from build123d import *

# Parameters (mm, degrees)
SKETCH1_R           = 16
BOSS_EXTRUDE1_DEPTH = 100
SKETCH2_R           = 3
BOSS_EXTRUDE2_DEPTH = 15
CIRPATTERN1_COUNT   = 4


with BuildPart() as part:
    # Sketch1 → Boss-Extrude1 (new body)
    with BuildSketch(Plane.XY):
        Circle(SKETCH1_R)
    extrude(amount=BOSS_EXTRUDE1_DEPTH)

    # Sketch2 → Boss-Extrude2 (add)
    with BuildSketch(Plane.XY.offset(100)):
        Circle(SKETCH2_R)
    extrude(amount=BOSS_EXTRUDE2_DEPTH)

    # Sketch6 → M3.5x0.6 Tapped Hole1 (revolve, cut)
    with BuildSketch(Plane(origin=(0, 13, 100), x_dir=(0, -1, 0), z_dir=(1, 0, 0))):
        Polygon((0, 0), (0, 9.761247898), (1.45, 8.89), (1.45, 0), align=None)
    m3_5x0_6_tapped_hole1 = revolve(axis=Axis((0, 13, 106.35), (0, 0, -1)), mode=Mode.SUBTRACT)

    # CirPattern1: M3.5x0.6 Tapped Hole1 ×4 about axis
    cirpattern1_axis = Axis((0, 0, 0), (0, 0, 1))
    for i in range(1, CIRPATTERN1_COUNT):
        add(m3_5x0_6_tapped_hole1.rotate(cirpattern1_axis, i * 360 / CIRPATTERN1_COUNT), mode=Mode.SUBTRACT)


solid = part.part
Geometry: final body of the model. Coordinates: model frame, mm. A direction names the side the tool comes from. Coordinates: 2 decimals unless noted, no trailing zeros. Loops run counter-clockwise (first coordinate to the right, second up) from the corner with the lowest first, then second, coordinate; pieces in that order, holes last. Notation, with made-up numbers: (-39, -30.5) - (-25, -30.5) arc R19 ccw to (-25, -26.5) - close; hole circle Ø6 at (-25.5, -22). An arc over 180 degrees is marked (long way). Put each result on its own line as item: value. Start each with the question number.
Q1. Cut plane D-D, the plane z = 105.5. Return loops of the section in (x, y), and give its area (3 significant figures).
Q2. Line query: line 1 (Z direction, x = -10, y = -2); line 2 (Y direction, x = 13, z = 94.5). Output: solid intervals per line, ascending.
Q3. Pull-direction query (X, two-part tool) for faces 1 (the conical face through (-13.25, -0.01, 90.39)), 2 (the cylindrical face through (-3, 0, 107)), 3 (the flat face through (0, 0, 0)); classes: released by +X, released by -X, zero draft, split by the parting line, or undercut.
Q4. Cut plane A-A, the plane z = 35. Return loops of the section in (x, y).
Q5. Cut plane B-B, the plane x = 6. Return loops of the section in (y, z).
Q6. Cut plane C-C, the plane y = 5. Return loops of the section in (x, z), and give its area (3 significant figures).
Q7. Pin query (flat end, axial travel): pin 1 Ø10 at (y, z) = (8.5, 29.5) entering from -X; pin 2 Ø8 at (x, z) = (-11.5, 96.5) entering from -Y; pin 3 Ø5 at (y, z) = (-10.5, 87.5) entering from -X. Return the tip coordinate at first contact, or that it passes through.
Q8. Set-up query: faces 4 (the cylindrical face through (0.98, -14.07, 95.62)), 5 (the flat face through (0, 0, 115)). Return all of +Z, -Z, +X, -X, +Y, -Y with unobstructed straight access to the full face (end or side cutting, diameter ignored); none if empty.
Filled sheet:
1. outline: circle Ø6 at (0, 0)
1. area: 28.3 mm²
2. line 1: 0 to 100
2. line 2: -9.33 to -1.45, 1.45 to 9.33
3. face 1: undercut
3. face 2: split by the parting line
3. face 3: zero draft
4. outline: circle Ø32 at (0, 0)
5. outline: (-14.83, 0) - (14.83, 0) - (14.83, 100) - (-14.83, 100) - close
6. outline: (-15.2, 0) - (15.2, 0) - (15.2, 100) - (-15.2, 100) - close
6. area: 3,040 mm²
7. pin 1: x = -15.61
7. pin 2: y = -14.13
7. pin 3: x = -13.86
8. face 4: +Z
8. face 5: +Z, +X, -X, +Y, -Y
